```python
from build123d import *

# Parameters (mm, degrees)
MODULE_START                                    = 25.2
SKETCH_1_W                                      = 39.2
SKETCH_1_H                                      = 27.8
MODULE_PCB_DEPTH                                = 1.2
BACKLIGHT_START                                 = 26.4
SKETCH_2_W                                      = 29.22
SKETCH_2_H                                      = 25.8
BACKLIGHT_FRAME_DEPTH                           = 1
GLASS_START                                     = 27.4
SKETCH_3_W                                      = 29.22
SKETCH_3_H                                      = 25.8
GLASS_DEPTH                                     = 0.6
F_7_PIN_START                                   = 22.66
SKETCH_4_W                                      = 2.54
SKETCH_4_H                                      = 17.78
F_7_PIN_HEADER_PLASTIC_ON_THE_MODULE_BACK_DEPTH = 2.54
SKETCH_5_R                                      = 1
CORNER_HOLES_DEPTH                              = 82.935157289
M2_START                                        = 23.9
SKETCH_6_R                                      = 1.9
M2_SCREW_HEAD_DEPTH                             = 1.3
EXTRUDE_START                                   = 23.9
SKETCH_7_R                                      = 1.9
EXTRUDE_6_DEPTH                                 = 1.3
SKETCH_8_R                                      = 1.9
EXTRUDE_7_DEPTH                                 = 1.3
SKETCH_9_R                                      = 1.9
EXTRUDE_8_DEPTH                                 = 1.3


with BuildPart() as part:
    # 草圖1 → module PCB (new body)
    with BuildSketch(Plane.XY.offset(MODULE_START)):
        with Locations((30, 45)):
            Rectangle(SKETCH_1_W, SKETCH_1_H)
    extrude(amount=MODULE_PCB_DEPTH)

    # 草圖2 → backlight frame (add)
    with BuildSketch(Plane.XY.offset(BACKLIGHT_START)):
        with Locations((30, 45)):
            Rectangle(SKETCH_2_W, SKETCH_2_H)
    extrude(amount=BACKLIGHT_FRAME_DEPTH)

    # 草圖3 → glass (add)
    with BuildSketch(Plane.XY.offset(GLASS_START)):
        with Locations((30, 45)):
            Rectangle(SKETCH_3_W, SKETCH_3_H)
    extrude(amount=GLASS_DEPTH)

    # 草圖4 → 7-pin header plastic on the module back (add)
    with BuildSketch(Plane.XY.offset(F_7_PIN_START)):
        with Locations((12.9, 45)):
            Rectangle(SKETCH_4_W, SKETCH_4_H)
    extrude(amount=F_7_PIN_HEADER_PLASTIC_ON_THE_MODULE_BACK_DEPTH)

    # 草圖5 → corner holes (cut, through all)
    with BuildSketch(Plane.XY):
        with Locations((12.9, 33.6)):
            Circle(SKETCH_5_R)
        with Locations((12.9, 56.4)):
            Circle(SKETCH_5_R)
        with Locations((47.1, 33.6)):
            Circle(SKETCH_5_R)
        with Locations((47.1, 56.4)):
            Circle(SKETCH_5_R)
    extrude(amount=CORNER_HOLES_DEPTH, mode=Mode.SUBTRACT)

    # 草圖6 → M2 screw head (add)
    with BuildSketch(Plane.XY.offset(M2_START)):
        with Locations((12.9, 33.6)):
            Circle(SKETCH_6_R)
    extrude(amount=M2_SCREW_HEAD_DEPTH)

    # 草圖7 → 填料-伸長6 (add)
    with BuildSketch(Plane.XY.offset(EXTRUDE_START)):
        with Locations((12.9, 56.4)):
            Circle(SKETCH_7_R)
    extrude(amount=EXTRUDE_6_DEPTH)

    # 草圖8 → 填料-伸長7 (add)
    with BuildSketch(Plane.XY.offset(EXTRUDE_START)):
        with Locations((47.1, 33.6)):
            Circle(SKETCH_8_R)
    extrude(amount=EXTRUDE_7_DEPTH)

    # 草圖9 → 填料-伸長8 (add)
    with BuildSketch(Plane.XY.offset(EXTRUDE_START)):
        with Locations((47.1, 56.4)):
            Circle(SKETCH_9_R)
    extrude(amount=EXTRUDE_8_DEPTH)


solid = part.part
```
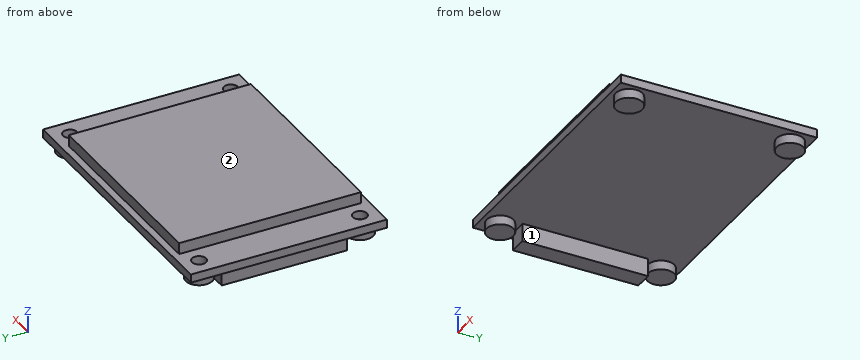
Read the model definition and answer for the solid it produces. Units are mm, in the model's axes. Face numbers are marked on the shaded views. Give positions to 0.01 mm unless a question says otherwise; leave off trailing zeros. Loops run counter-clockwise (first coordinate to the right, second up) from the corner with the lowest first, then second, coordinate; pieces in that order, holes last.
Item 1: The mould has two halves that part along Y. Classify the marked faces 1 and 2: released by +Y, released by -Y, zero draft, split by the parting line, or undercut.
Item 2: The part is cut by section B-B (x = 44). Write down the section's boundary in (y, z).
Item 3: The part is cut by section A-A (z = 24.4). Write down the section's boundary in (x, y), and give its area (3 significant figures).
Item 4: Each of these flat-tipped pins is pushed along its axis until it touches: pin 1 Ø0.6 at (x, y) = (47.5, 56.5) entering from +Z; pin 2 Ø1.8 at (x, y) = (12.9, 56.4) entering from -Z; pin 3 Ø4 at (x, y) = (24, 42.5) entering from -Z. Where does it stop, or does it pass through?
Item 5: The part is cut by section C-C (y = 56.4). Write down the section's boundary in (x, z), and give its area (3 significant figures).
Item 6: Find the intervals of material crossed by line 1 along Y through (x, z) = (12.9, 25.65); line 2 along X through (y, z) = (56.4, 26.05); line 3 along Y through (x, z) = (13, 24.5), in increasing order.
Item 7: The part is cut by section D-D (x = 12.9). Write down the section's boundary in (y, z), and give its area (3 significant figures).
Taken from the geometry:
1. face 1: undercut
1. face 2: zero draft
2. outline: (31.1, 25.2) - (58.9, 25.2) - (58.9, 26.4) - (57.9, 26.4) - (57.9, 28) - (32.1, 28) - (32.1, 26.4) - (31.1, 26.4) - close
3. outline: circle Ø3.8 at (12.9, 33.6); circle Ø3.8 at (12.9, 56.4); (11.63, 36.11) - (14.17, 36.11) - (14.17, 53.89) - (11.63, 53.89) - close; circle Ø3.8 at (47.1, 33.6); circle Ø3.8 at (47.1, 56.4)
3. area: 90.5 mm2
4. pin 1: stops at z = 25.2
4. pin 2: stops at z = 23.9
4. pin 3: stops at z = 25.2
5. outline: (10.4, 25.2) - (11, 25.2) - (11, 23.9) - (14.8, 23.9) - (14.8, 25.2) - (45.2, 25.2) - (45.2, 23.9) - (49, 23.9) - (49, 25.2) - (49.6, 25.2) - (49.6, 26.4) - (48.1, 26.4) - (48.1, 25.2) - (46.1, 25.2) - (46.1, 26.4) - (44.61, 26.4) - (44.61, 28) - (15.39, 28) - (15.39, 26.4) - (13.9, 26.4) - (13.9, 25.2) - (11.9, 25.2) - (11.9, 26.4) - (10.4, 26.4) - close
5. area: 98.9 mm2
6. line 1: y = 31.1 to 32.6, 34.6 to 55.4, 57.4 to 58.9
6. line 2: x = 10.4 to 11.9, 13.9 to 46.1, 48.1 to 49.6
6. line 3: y = 31.7 to 35.5, 36.11 to 53.89, 54.5 to 58.3
7. outline: (31.1, 25.2) - (31.7, 25.2) - (31.7, 23.9) - (35.5, 23.9) - (35.5, 25.2) - (36.11, 25.2) - (36.11, 22.66) - (53.89, 22.66) - (53.89, 25.2) - (54.5, 25.2) - (54.5, 23.9) - (58.3, 23.9) - (58.3, 25.2) - (58.9, 25.2) - (58.9, 26.4) - (57.4, 26.4) - (57.4, 25.2) - (55.4, 25.2) - (55.4, 26.4) - (34.6, 26.4) - (34.6, 25.2) - (32.6, 25.2) - (32.6, 26.4) - (31.1, 26.4) - close
7. area: 83.6 mm2
